```python
from build123d import *

# Parameters (mm, degrees)
SKETCH1_W               = 152.4
SKETCH1_H               = 101.6
BOSS_EXTRUDE1_DEPTH     = 19.05
CUT_EXTRUDE1_DEPTH      = 185.15
CUT_EXTRUDE1_DEPTH_BACK = 185.15
BOSS_EXTRUDE2_DEPTH     = 12.7


with BuildPart() as part:
    # Sketch1 → Boss-Extrude1 (new body)
    with BuildSketch(Plane.XY):
        with Locations((76.2, 50.8)):
            Rectangle(SKETCH1_W, SKETCH1_H)
    extrude(amount=BOSS_EXTRUDE1_DEPTH)

    # Sketch4 → Cut-Extrude1 (cut, two sides: drawn at the far end of the back side and taken through both)
    with BuildSketch(Plane.XY.offset(19.05).offset(-CUT_EXTRUDE1_DEPTH_BACK)):
        with BuildLine():
            ThreePointArc((85.725, 50.8), (82.935192091, 57.535192091), (76.2, 60.325))
            Line((76.2, 60.325), (76.2, 50.8))
            Line((76.2, 50.8), (85.725, 50.8))
        make_face()
        with BuildLine():
            Line((152.4, 50.8), (152.4, 101.6))
            Line((152.4, 101.6), (76.2, 101.6))
            Line((76.2, 101.6), (76.2, 60.325))
            ThreePointArc((76.2, 60.325), (82.935192091, 57.535192091), (85.725, 50.8))
            Line((85.725, 50.8), (152.4, 50.8))
        make_face()
    extrude(amount=CUT_EXTRUDE1_DEPTH + CUT_EXTRUDE1_DEPTH_BACK, mode=Mode.SUBTRACT)

    # Sketch4_4 → Boss-Extrude2 (add)
    with BuildSketch(Plane.XY.offset(19.05)):
        with BuildLine():
            Line((76.2, 50.8), (76.2, 60.325))
            ThreePointArc((76.2, 60.325), (69.464807909, 44.064807909), (85.725, 50.8))
            Line((85.725, 50.8), (76.2, 50.8))
        make_face()
    extrude(amount=BOSS_EXTRUDE2_DEPTH)


solid = part.part
```
Can you work these out from the model? Positions are in its coordinate system, mm. A direction names the side the tool comes from. Round coordinates to 2 decimals unless told otherwise and drop trailing zeros. Order: outer loops, then holes, each group sorted by start corner. A loop starts at its lowest first (then second) coordinate and runs counter-clockwise, first axis right, second up. Notation, with made-up numbers: (-8.75, 34) -> (10.25, 34) arc R26 cw to (10.25, 57) -> close; hole circle Ø5 at (46, -36.5). An arc over 180 degrees is marked (long way). Return JSON: item names as keys, results as strings. Group by question number.
1. Will these pins go through, and if not, where does the flat tip stop? pin 1 (5 mm diameter, centred on x = 66.5, y = 36, fed in from +Z); pin 2 (4 mm diameter, centred on x = 95.5, z = 19, fed in from +Y); pin 3 (1.5 mm diameter, centred on y = 70.5, z = 17, fed in from +X).
2. I need wall thicknesses on line 1 (X direction, y = 50.5, z = 24); line 2 (Z direction, x = 12, y = 15.5); line 3 (X direction, y = 54.5, z = 4.5). Which ranges of each line are inside material? Lowest first, please. Write a range as [from, to].
3. If we section it at B-B, the plane y = 86.5: Write out the boundary of the cut face in (x, z).
4. If we section it at C-C, the plane x = 24: Write out the boundary of the cut face in (y, z), then the cut area to 3 significant figures.
5. If we section it at A-A, the plane z = 14: Write out the boundary of the cut face in (x, y), then the cut area to 3 significant figures.
6. Which directions (+Z, -Z, +X, -X, +Y, -Y) give clear straight access to the entire face, cutting with the end or side of a thin tool? Please do faces 1 (the face through (38, 101.6, 9)), 2 (the face through (115, 50.8, 9)), 3 (the face through (69.246, 44.291, 25.311)).
Output values:
{
 "1": {"pin 1": "z = 19.05", "pin 2": "y = 50.8", "pin 3": "x = 76.2"},
 "2": {"line 1": "[66.68, 85.72]", "line 2": "[0, 19.05]", "line 3": "[0, 76.2]"},
 "3": {"outline": "(0, 0) -> (76.2, 0) -> (76.2, 19.05) -> (0, 19.05) -> close"},
 "4": {"outline": "(0, 0) -> (101.6, 0) -> (101.6, 19.05) -> (0, 19.05) -> close", "area": "1,940 mm²"},
 "5": {"outline": "(0, 0) -> (152.4, 0) -> (152.4, 50.8) -> (76.2, 50.8) -> (76.2, 101.6) -> (0, 101.6) -> close", "area": "11,600 mm²"},
 "6": {"face 1": "+Z, -Z, +X, -X, +Y", "face 2": "+Z, -Z, +X, +Y", "face 3": "+Z"}
}
